from build123d import *

# Parameters (mm, degrees)
SKETCH_W          = 42.3
SKETCH_H          = 42.3
PAD_DEPTH         = 40
SKETCH001_R       = 11
PAD001_DEPTH      = 2
SKETCH002_R       = 2.5
PAD002_DEPTH      = 24
CHAMFER_SIZE      = 0.5
SKETCH003_W       = 0.5
SKETCH003_H       = 21
POCKET_DEPTH      = 21.151
POCKET_DEPTH_BACK = 21.151
SKETCH004_R       = 0.875
HOLE_DEPTH        = 3.474247
HOLE_TIPS_R       = 0.875
CHAMFER001_SIZE   = 5


with BuildPart() as part:
    # Sketch → Pad (new body)
    with BuildSketch(Plane.XY):
        Rectangle(SKETCH_W, SKETCH_H)
    extrude(amount=PAD_DEPTH)

    # Sketch001 (on Face6 of Pad) → Pad001 (join)
    with BuildSketch(Plane.XY.offset(40)):
        Circle(SKETCH001_R)
    extrude(amount=PAD001_DEPTH)

    # Sketch002 (on Face5 of Pad001) → Pad002 (join)
    with BuildSketch(Plane.XY.offset(40)):
        Circle(SKETCH002_R)
    extrude(amount=PAD002_DEPTH)

    # Chamfer
    chamfer_edges = [part.edges().sort_by_distance(p)[0] for p in [
        (-2.5, 0, 64),
    ]]
    chamfer(chamfer_edges, length=CHAMFER_SIZE)

    # Sketch003 → Pocket (cut, two sides)
    with BuildSketch(Plane.XZ) as pocket_sk:
        with Locations((2.25, 53.5)):
            Rectangle(SKETCH003_W, SKETCH003_H)
    extrude(amount=-POCKET_DEPTH, mode=Mode.SUBTRACT)
    extrude(pocket_sk.sketch, amount=POCKET_DEPTH_BACK, mode=Mode.SUBTRACT)

    # Sketch004 (on Face8 of Pocket) → Hole (cut)
    with BuildSketch(Plane.XY.offset(40)):
        with Locations((15.5, -15.5)):
            Circle(SKETCH004_R)
        with Locations((15.5, 15.5)):
            Circle(SKETCH004_R)
        with Locations((-15.5, 15.5)):
            Circle(SKETCH004_R)
        with Locations((-15.5, -15.5)):
            Circle(SKETCH004_R)
    extrude(amount=-HOLE_DEPTH, mode=Mode.SUBTRACT)

    # Hole tips → Hole tip 1 section 0
    with BuildSketch(Plane.XY.offset(36.525753), mode=Mode.PRIVATE) as hole_tip_1_s0:
        with Locations((15.5, -15.5)):
            Circle(HOLE_TIPS_R)
    loft([hole_tip_1_s0.sketch, Vertex(15.5, -15.5, 36)], mode=Mode.SUBTRACT)

    # Hole tips → Hole tip 2 section 0
    with BuildSketch(Plane.XY.offset(36.525753), mode=Mode.PRIVATE) as hole_tip_2_s0:
        with Locations((15.5, 15.5)):
            Circle(HOLE_TIPS_R)
    loft([hole_tip_2_s0.sketch, Vertex(15.5, 15.5, 36)], mode=Mode.SUBTRACT)

    # Hole tips → Hole tip 3 section 0
    with BuildSketch(Plane.XY.offset(36.525753), mode=Mode.PRIVATE) as hole_tip_3_s0:
        with Locations((-15.5, 15.5)):
            Circle(HOLE_TIPS_R)
    loft([hole_tip_3_s0.sketch, Vertex(-15.5, 15.5, 36)], mode=Mode.SUBTRACT)

    # Hole tips → Hole tip 4 section 0
    with BuildSketch(Plane.XY.offset(36.525753), mode=Mode.PRIVATE) as hole_tip_4_s0:
        with Locations((-15.5, -15.5)):
            Circle(HOLE_TIPS_R)
    loft([hole_tip_4_s0.sketch, Vertex(-15.5, -15.5, 36)], mode=Mode.SUBTRACT)

    # Chamfer001
    chamfer001_edges = [part.edges().sort_by_distance(p)[0] for p in [
        (21.15, -21.15, 20),
        (21.15, 21.15, 20),
        (-21.15, -21.15, 20),
        (-21.15, 21.15, 20),
    ]]
    chamfer(chamfer001_edges, length=CHAMFER001_SIZE)


solid = part.part
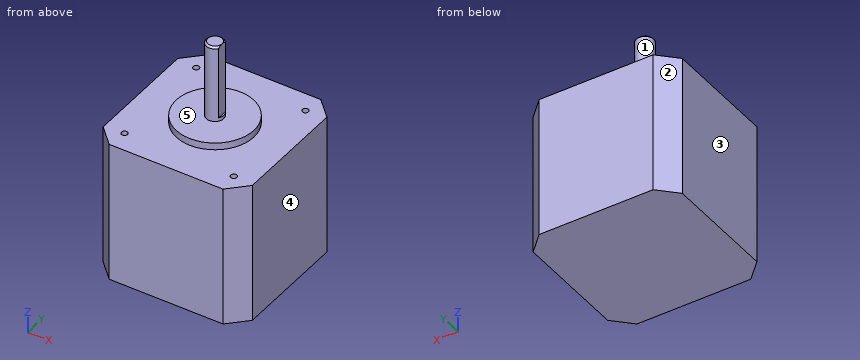
Source: CAD feature listing. Evaluate the final solid. Frame: model axes, mm. Face numbers are marked on the shaded views. A direction names the side the tool comes from. Give positions to 0.01 mm unless a question says otherwise; leave off trailing zeros. Loops run counter-clockwise (first coordinate to the right, second up) from the corner with the lowest first, then second, coordinate; pieces in that order, holes last. Notation, with made-up numbers: (13, 81) -> (48, 81) arc R11 cw to (48, 99) -> close; hole circle Ø9 at (39, 73.5). An arc over 180 degrees is marked (long way). Use a Markdown table: item, result. Add a question column.
1) Section query B-B, the plane x = 0. Return the cut outline in (y, z), then the cut area to 3 significant figures.
2) First-contact query: pin 1 (10 mm diameter, centred on x = -15.5, y = -9.5, fed in from -Z); pin 2 (2 mm diameter, centred on x = -15.5, y = 15.5, fed in from +Z); pin 3 (12 mm diameter, centred on x = -3, y = 11.5, fed in from +Z); pin 4 (1.1 mm diameter, centred on x = 15.5, y = 15.5, fed in from +Z). Flat tips, straight axial feed; report the tip coordinate or a pass-through.
3) Reachability of the marked faces 1 and 2 from +Z, -Z, +X, -X, +Y, -Y: full face, straight path, thin tool, end or side. Return the list, or none.
4) Line query: line 1 along Y through (x, z) = (-15.5, 38.45) (3 decimals); line 2 along Y through (x, z) = (15, 38). Output: solid intervals per line, ascending. Write a range as [from, to].
5) Section query D-D, the plane y = -13.5. Return the cut outline in (x, z).
6) Section query C-C, the plane y = 3.5. Return the cut outline in (x, z), then the cut area to 3 significant figures.
7) Section query A-A, the plane z = 31.5. Return the cut outline in (x, y), then the cut area to 3 significant figures.
8) Pull-direction query (X, two-part tool) for the marked faces 3, 4 and 5; classes: +X half, -X half, draft (parallel to the pull), parting line (faces both ways), or undercut.
Numbers:
| question | item | result |
|---|---|---|
| 1 | outline | (-21.15, 0) -> (21.15, 0) -> (21.15, 40) -> (11, 40) -> (11, 42) -> (2.5, 42) -> (2.5, 63.5) -> (2, 64) -> (-2, 64) -> (-2.5, 63.5) -> (-2.5, 42) -> (-11, 42) -> (-11, 40) -> (-21.15, 40) -> close |
| 1 | area | 1,850 mm2 |
| 2 | pin 1 | stops at z = 0 |
| 2 | pin 2 | stops at z = 40 |
| 2 | pin 3 | stops at z = 42 |
| 2 | pin 4 | stops at z = 36.33 |
| 3 | face 1 | +Z |
| 3 | face 2 | +Z, -Z, -X, +Y |
| 4 | line 1 | y = [-21.15, -16.375], [-14.625, 14.625], [16.375, 21.15] |
| 4 | line 2 | y = [-21.15, -16.22], [-14.78, 14.78], [16.22, 21.15] |
| 5 | outline | (-21.15, 0) -> (21.15, 0) -> (21.15, 40) -> (-21.15, 40) -> close |
| 6 | outline | (-21.15, 0) -> (21.15, 0) -> (21.15, 40) -> (10.43, 40) -> (10.43, 42) -> (-10.43, 42) -> (-10.43, 40) -> (-21.15, 40) -> close |
| 6 | area | 1,730 mm2 |
| 7 | outline | (-21.15, -16.15) -> (-16.15, -21.15) -> (16.15, -21.15) -> (21.15, -16.15) -> (21.15, 16.15) -> (16.15, 21.15) -> (-16.15, 21.15) -> (-21.15, 16.15) -> close |
| 7 | area | 1,740 mm2 |
| 8 | face 3 | -X half |
| 8 | face 4 | +X half |
| 8 | face 5 | draft |
